```python
from build123d import *

# Parameters (mm, degrees)
SKETCH_1_W          = 8
SKETCH_1_H          = 100
EXTRUDE_1_DEPTH     = 2.95
SKETCH_2_R          = 0.7
CUT_EXTRUDE_1_DEPTH = 101.362854184
SKETCH_2_3_R        = 1
CUT_EXTRUDE_2_DEPTH = 1.5


with BuildPart() as part:
    # Sketch 1 → Extrude 1 (new body)
    with BuildSketch(Plane(origin=(0, 0, 0), x_dir=(1, 0, 0), z_dir=(0, 1, 0))):
        with Locations((4, -50)):
            Rectangle(SKETCH_1_W, SKETCH_1_H)
    extrude(amount=EXTRUDE_1_DEPTH)

    # Sketch 2 → Cut-Extrude 1 (cut, through all)
    with BuildSketch(Plane(origin=(0, 2.95, 0), x_dir=(1, 0, 0), z_dir=(0, 1, 0))):
        with Locations(Location((4, -8, 0), (0, 0, 270))):
            Circle(SKETCH_2_R)
        with Locations(Location((4, -2, 0), (0, 0, 270))):
            Circle(SKETCH_2_R)
        with Locations(Location((4, -98, 0), (0, 0, 270))):
            Circle(SKETCH_2_R)
        with Locations(Location((4, -92, 0), (0, 0, 270))):
            Circle(SKETCH_2_R)
    extrude(amount=-CUT_EXTRUDE_1_DEPTH, mode=Mode.SUBTRACT)

    # Sketch 2_3 → Cut-Extrude 2 (cut)
    with BuildSketch(Plane(origin=(0, 2.95, 0), x_dir=(1, 0, 0), z_dir=(0, 1, 0))):
        with Locations(Location((4, -8, 0), (0, 0, 270))):
            Circle(SKETCH_2_3_R)
        with Locations(Location((4, -2, 0), (0, 0, 270))):
            Circle(SKETCH_2_3_R)
        with Locations(Location((4, -98, 0), (0, 0, 270))):
            Circle(SKETCH_2_3_R)
        with Locations(Location((4, -92, 0), (0, 0, 270))):
            Circle(SKETCH_2_3_R)
    extrude(amount=-CUT_EXTRUDE_2_DEPTH, mode=Mode.SUBTRACT)


solid = part.part
```
Build history of the part. All positions in model axes, mm. A direction names the side the tool comes from. Round coordinates to 2 decimals unless told otherwise and drop trailing zeros. Write each loop counter-clockwise with the first axis right and the second up, starting at its lowest first coordinate (ties: lowest second). Pieces come first, ordered by that corner, then holes.
1) 3-axis set-ups, long thin cutter, end or side, ignore diameter. For faces 1 (the cylindrical face through (5, 2, 8)), 2 (the flat face through (4, 0, 49)): which of +Z, -Z, +X, -X, +Y, -Y reach the whole face in a straight line?
2) Drill centre lines: probe 1 along X at (y, z) = (2.1, 2); probe 2 along Z at (x, y) = (4.25, 0.95). Where is each one in solid material? Low to high.
3) Band-saw the part on A-A, the plane y = 1.9. List the corners of the cut face in (x, z).
4) Mould opens along Z. For faces 3 (the flat face through (4, 2.95, 49)), 4 (the cylindrical face through (4, 2, 97)), 5 (the flat face through (4, 1, 100)) say: +Z half, -Z half, draft (parallel to the pull), parting line (faces both ways), or undercut.
5) Pin check, flat tip, straight feed: pin 1 (0.6 mm diameter, centred on x = 4, z = 98.5, fed in from +Y). Stop position of the tip, or through.
Ans:
1. face 1: +Y
1. face 2: +Z, -Z, +X, -X, -Y
2. probe 1: x = 0 to 3, 5 to 8
2. probe 2: z = 0 to 1.35, 2.65 to 7.35, 8.65 to 91.35, 92.65 to 97.35, 98.65 to 100
3. outline: (0, 0) - (8, 0) - (8, 100) - (0, 100) - close; hole circle Ø2 at (4, 2); hole circle Ø2 at (4, 8); hole circle Ø2 at (4, 92); hole circle Ø2 at (4, 98)
4. face 3: draft
4. face 4: undercut
4. face 5: +Z half
5. pin 1: stops at y = 1.45
